Autodesk Inventor part; units mm, degrees
ref_plane "YZ Plane" through (0, 0, 0) normal (1, 0, 0) x (0, 1, 0)
ref_plane "XZ Plane" through (0, 0, 0) normal (0, 1, 0) x (-1, 0, 0)
ref_plane "XY Plane" through (0, 0, 0) normal (0, 0, 1) x (1, 0, 0)
sketch "Sketch1" plane through (0, 0, 0) normal (1, 0, 0) x (0, 1, 0)
  circle A0 centre (0, 0) radius 3.25
  circle A1 centre (0, 0) radius 2
  dimension "d0" = 6.5
  dimension "d1" = 4
extrude "Extrusion1" add sketch "Sketch1" along normal blind 5 contours A0 | A1
sketch "Sketch2" plane through (5, 0, 0) normal (1, 0, 0) x (0, 0, -1)
  circle A0 centre (0, 0) radius 2
  dimension "d4" = 4
extrude "Extrusion2" add sketch "Sketch2" along normal blind 70
sketch "Sketch3" plane through (0, 0, 0) normal (-1, 0, 0) x (0, 0, 1)
  circle A0 centre (0, 0) radius 2
  line L0 (2, -1.1547) -> (0, -2.3094)
  line L1 (0, -2.3094) -> (-2, -1.1547)
  line L2 (-2, -1.1547) -> (-2, 1.1547)
  line L3 (-2, 1.1547) -> (0, 2.3094)
  line L4 (0, 2.3094) -> (2, 1.1547)
  line L5 (2, 1.1547) -> (2, -1.1547)
  point P0 (2, 0)
extrude "Extrusion3" cut sketch "Sketch3" against normal blind 3.5
thread "Thread1"
fillet "Fillet1" radius 0.5 3 edges at (5, 0, 2) (0, -3.25, 0) (75, 0, 2)
sketch "Sketch4" plane through (75, 0, 0) normal (1, 0, 0) x (0, 0, -1)
  line L0 (-7.7054, 6.4284) -> (8.1646, 6.4284)
  line L1 (8.1646, 6.4284) -> (8.1646, -6.8875)
  line L2 (8.1646, -6.8875) -> (-7.7054, -6.8875)
  line L3 (-7.7054, -6.8875) -> (-7.7054, 6.4284)
  point P0 (0, 0)
extrude "Extrusion4" cut sketch "Sketch4" against normal blind 5
fillet "Fillet2" radius 0.3 1 edges at (70, 0, 2)
properties part number "m4x70_example" material "Stainless Steel"
Design review of the part built by this model. Coordinates are the model's own, in mm. A direction names the side the tool comes from. Give positions to 0.01 mm unless a question says otherwise; leave off trailing zeros. Loops run counter-clockwise (first coordinate to the right, second up) from the corner with the lowest first, then second, coordinate; pieces in that order, holes last. Notation, with made-up numbers: M -29.75,-28.75 L -6.75,-28.75 A29 cw -6.75,-6.75 Z; hole C 73.5,-1.75 d10. An arc over 180 degrees is marked long. Answer as a JSON object with one key per item and string values.
Item 1: Wall thickness on line 1 along X through (y, z) = (1, 1); line 2 along X through (y, z) = (-0.5, 2.5); line 3 along Z through (x, y) = (6, 0): over which ranges is each line inside the solid? List them lowest first.
Output values:
{"line 1": "x = 3.5 to 70", "line 2": "x = 0 to 5", "line 3": "z = -2 to 2"}
Item 2: Machinability: for faces 4 (the face through (2, 0, 2)), 5 (the face through (0, 2, -1)), 6 (the face through (5, 2, -2)), which of the approach directions +Z, -Z, +X, -X, +Y, -Y give a long, thin tool a straight path to every point of the face, cutting with its end or side? Answer none if there is none.
Output values:
{"face 4": "-X", "face 5": "+Z, -Z, -X, +Y, -Y", "face 6": "+X"}
Item 3: Mouldability with a two-part tool opening along Z and no side actions: class faces 1 (the face through (70, 0, 0)), 2 (the face through (2, 0, -2)), 3 (the face through (37, 2, 0)) as pulls with the +Z half, pulls with the -Z half, needs draft (parallel to the pull), parting line crosses it, or undercut.
Output values:
{"face 1": "needs draft", "face 2": "undercut", "face 3": "parting line crosses it"}
Item 4: We need section A-A (y = 0). State the section outline as (x, z) points, and give its area (3 significant figures).
Output values:
{"outline": "M 0,-2.75 A0.5 ccw 0.5,-3.25 L 5,-3.25 L 5,-2.5 A0.5 cw 5.5,-2 L 69.7,-2 A0.3 ccw 70,-1.7 L 70,1.7 A0.3 ccw 69.7,2 L 5.5,2 A0.5 cw 5,2.5 L 5,3.25 L 0.5,3.25 A0.5 ccw 0,2.75 L 0,2 L 3.5,2 L 3.5,-2 L 0,-2 Z", "area": "278 mm2"}
Item 5: We need section B-B (x = 40). State the section outline as (y, z) points, and give its area (3 significant figures).
Output values:
{"outline": "C 0,0 d4", "area": "12.6 mm2"}
Item 6: For P1, Ø1.5, axis at x = 38, z = 0.5, coming from the -Y side; P2, Ø1, axis at x = 46, y = -0.5, coming from the -Z side; P3, Ø2, axis at y = 0, z = -0.5, coming from the -X side, all flat-tipped, find the tip position at first contact; note any pin that passes through.
Output values:
{"P1": "stops at y = -2", "P2": "stops at z = -2", "P3": "stops at x = 3.5"}
